Read the model definition and answer for the solid it produces. Units are mm, in the model's axes. A direction names the side the tool comes from. Give positions to 0.01 mm unless a question says otherwise; leave off trailing zeros. Order: outer loops, then holes, each group sorted by start corner. A loop starts at its lowest first (then second) coordinate and runs counter-clockwise, first axis right, second up. Notation, with made-up numbers: (-9.5, 29) - (21.5, 29) arc R21 ccw to (21.5, 35) - close; hole circle Ø7 at (60.25, -18.5). An arc over 180 degrees is marked (long way). Write item = value, one per line.
```python
from build123d import *

# Parameters (mm, degrees)
F1_DEPTH = 5.842
F2_DEPTH = 3.81
F3_DEPTH = 2.032
F5_DEPTH = 0.508


with BuildPart() as f1:
    # F0 (on Top) → F1 (new body)
    with BuildSketch(Plane.XY):
        with BuildLine():
            ThreePointArc((3.175, 0), (0, 3.175), (-3.175, 0))
            ThreePointArc((-3.175, 0), (0, -3.175), (3.175, 0))
        make_face()
        with BuildLine():
            Line((-8.469026, -3.167854), (-8.982779, -3.167854))
            ThreePointArc((-8.982779, -3.167854), (-5.502355, -7.774942), (0, -9.525))
            ThreePointArc((0, -9.525), (9.525, 0), (0, 9.525))
            ThreePointArc((0, 9.525), (-5.499261, 7.77713), (-8.980256, 3.175))
            Line((-8.980256, 3.175), (-8.469026, 3.175))
            Line((-8.469026, 3.175), (-8.469026, 0))
            Line((-8.469026, 0), (-8.469026, -3.167854))
        make_face()
        with BuildLine():
            ThreePointArc((3.175, 0), (0, -3.175), (-3.175, 0))
            ThreePointArc((-3.175, 0), (0, 3.175), (3.175, 0))
        make_face(mode=Mode.SUBTRACT)
        with BuildLine():
            ThreePointArc((0, -9.525), (-5.502355, -7.774942), (-8.982779, -3.167854))
            Line((-8.982779, -3.167854), (-22.0853, -3.167854))
            Line((-22.0853, -3.167854), (-18.415, -9.525))
            Line((-18.415, -9.525), (-12.065, -9.525))
            Line((-12.065, -9.525), (-9.525, -9.525))
            Line((-9.525, -9.525), (0, -9.525))
        make_face()
        with BuildLine():
            ThreePointArc((-8.980256, 3.175), (-5.499261, 7.77713), (0, 9.525))
            Line((0, 9.525), (-9.525, 9.525))
            Line((-9.525, 9.525), (-12.065, 9.525))
            Line((-12.065, 9.525), (-18.415, 9.525))
            Line((-18.415, 9.525), (-22.081174, 3.175))
            Line((-22.081174, 3.175), (-8.980256, 3.175))
        make_face()
    extrude(amount=F1_DEPTH)

    # F0 (on Top) → F2 (join)
    with BuildSketch(Plane.XY):
        with BuildLine():
            ThreePointArc((3.175, 0), (0, 3.175), (-3.175, 0))
            ThreePointArc((-3.175, 0), (0, -3.175), (3.175, 0))
        make_face()
    extrude(amount=F2_DEPTH)

    # F0 (on Top) → F3 (cut)
    with BuildSketch(Plane.XY):
        with BuildLine():
            ThreePointArc((3.175, 0), (0, 3.175), (-3.175, 0))
            ThreePointArc((-3.175, 0), (0, -3.175), (3.175, 0))
        make_face()
    extrude(amount=F3_DEPTH, mode=Mode.SUBTRACT)

    # F4 (on face) → F5 (join)
    with BuildSketch(Plane(origin=(0, -3.167854, 0), x_dir=(-1, 0, 0), z_dir=(0, 1, 0))):
        with BuildLine():
            ThreePointArc((16.670343, 5.588), (13.876343, 2.794), (16.670343, 0))
            Line((16.670343, 0), (16.670343, 5.588))
        make_face()
        with BuildLine():
            Line((16.670343, 5.588), (16.670343, 0))
            ThreePointArc((16.670343, 0), (18.645999, 0.818344), (19.464343, 2.794))
            ThreePointArc((19.464343, 2.794), (18.645999, 4.769656), (16.670343, 5.588))
        make_face()
    extrude(amount=F5_DEPTH)


solid = f1.part
```
1. Determine the mould class of faces 1 (the face through (-7, 0, 5.842)), 2 (the face through (0, 0, 2.032)), 3 (the face through (-20.222, 6.394, 2.88)) for opening direction X: +X half, -X half, draft (parallel to the pull), parting line (faces both ways), or undercut.
Recorded:
face_1 = draft
face_2 = undercut
face_3 = -X half
2. Straight lines are drawn through the part: L1, parallel to X at y = 0, z = 4.7 (3 decimals); L2, parallel to Y at x = -11, z = 0.3 (3 decimals); L3, parallel to Y at x = -2, z = 4 (3 decimals). For each, find the intervals that lie inside material, in ascending order. Write a range as [from, to].
Recorded:
L1 = [-8.469, -3.175], [3.175, 9.525]
L2 = [-9.525, -3.168], [3.175, 9.525]
L3 = [-9.525, -2.466], [2.466, 9.525]
3. Section D-D (x = 0.5) is taken. Determine the outline of the cut face in (y, z).
Recorded:
outline = (-9.51, 0) - (-3.14, 0) - (-3.14, 2.03) - (3.14, 2.03) - (3.14, 0) - (9.51, 0) - (9.51, 5.84) - (3.14, 5.84) - (3.14, 3.81) - (-3.14, 3.81) - (-3.14, 5.84) - (-9.51, 5.84) - close
4. For faces 4 (the face through (0, 0, 3.81)), 5 (the face through (-17, -2.66, 3)), 6 (the face through (-20.276, -6.302, 2.88)), 7 (the face through (-3.03, -0.95, 1)), determine the directions among +Z, -Z, +X, -X, +Y, -Y from which every point of the face is accessible in a straight line to the end or side of a thin tool.
Recorded:
face_4 = +Z
face_5 = +Z, -Z, -X
face_6 = +Z, -Z, -X, -Y
face_7 = -Z
5. Section A-A (x = -9.5) is taken. Determine the outline of the cut face in (y, z) (3 decimals).
Recorded:
outline = (-9.525, 0) - (-3.168, 0) - (-3.168, 5.842) - (-9.525, 5.842) - close; (3.175, 0) - (9.525, 0) - (9.525, 5.842) - (3.175, 5.842) - close
6. Section C-C (y = 0) is taken. Determine the outline of the cut face in (x, z) (3 decimals), and give its area (3 significant figures).
Recorded:
outline = (-8.469, 0) - (-3.175, 0) - (-3.175, 2.032) - (3.175, 2.032) - (3.175, 0) - (9.525, 0) - (9.525, 5.842) - (3.175, 5.842) - (3.175, 3.81) - (-3.175, 3.81) - (-3.175, 5.842) - (-8.469, 5.842) - close
area = 79.3 mm^2
7. Flat-ended cylindrical pins translate along their axes: pin 1 (1.9 mm diameter, centred on x = -1, y = -1, fed in from +Z); pin 2 (1.5 mm diameter, centred on y = 4, z = 5, fed in from -X); pin 3 (3 mm diameter, centred on x = -1, y = -0.5, fed in from -Z). Find the tip coordinate at first contact, or state that the pin passes through.
Recorded:
pin_1 = 3.81
pin_2 = -22.04
pin_3 = 2.03
8. Section B-B (z = 0.55) is taken. Determine the outline of the cut face in (x, y) (3 decimals).
Recorded:
outline = (-22.085, -3.168) - (-18.415, -9.525) - (0, -9.525) arc R9.525 ccw to (0, 9.525) - (-18.415, 9.525) - (-22.081, 3.175) - (-8.469, 3.175) - (-8.469, -3.168) - (-15.006, -3.168) - (-15.006, -2.66) - (-18.335, -2.66) - (-18.335, -3.168) - close; hole circle Ø6.35 at (0, 0)
